Here's how the part is built. I have some questions about the finished solid (model axes, mm). Face numbers are marked on the shaded views. A direction names the side the tool comes from. Give positions to 0.01 mm unless a question says otherwise; leave off trailing zeros. Loops run counter-clockwise (first coordinate to the right, second up) from the corner with the lowest first, then second, coordinate; pieces in that order, holes last. Notation, with made-up numbers: M -31.5,-37 L 22.5,-37 A25 cw 22.5,-7 Z; hole C 13.5,44 d3. An arc over 180 degrees is marked long. Answer as CSV lines item,"result". Start each with the question number.
Item 1: If I drill on line 1 along X through (y, z) = (0, -20.5); line 2 along Z through (x, y) = (10.5, -3.5); line 3 along Z through (x, y) = (4, 6.5), over which ranges is the centre line in solid material (lowest first)? Write a range as from..to.
Item 2: I want a section at B-B on z = -4. List the corners of the cut face in (x, y) for me, plus the area to 3 significant figures.
Item 3: I want a section at C-C on x = 13. List the corners of the cut face in (y, z) for me.
Item 4: I want a section at A-A on y = 0. List the corners of the cut face in (x, z) for me.
Item 5: If we mould it in two halves opening along Y, with no side actions, what happens to the marked faces 1, 2, 3 and 4? For each: released by +Y, released by -Y, zero draft, split by the parting line, or undercut.
Item 6: For the marked faces 5, 6 and 7, which set-ups out of +Z, -Z, +X, -X, +Y, -Y let a thin tool reach every point of the face, with its end or its side?
Item 7: I want a section at D-D on z = 12.5. List the corners of the cut face in (x, y) for me, plus the area to 3 significant figures.
Item 8: Will these pins go through, and if not, where does the flat tip stop? P1, Ø4, axis at y = 19.05, z = 0, coming from the +X side; P2, Ø2, axis at x = 16, y = 0, coming from the +Z side; P3, Ø6, axis at x = 14, y = -6, coming from the +Z side; P4, Ø4, axis at y = 9, z = 7, coming from the -X side.
Autodesk Inventor part; units mm, degrees
ref_plane "YZ Plane" through (0, 0, 0) normal (1, 0, 0) x (0, 1, 0)
ref_plane "XZ Plane" through (0, 0, 0) normal (0, 1, 0) x (-1, 0, 0)
ref_plane "XY Plane" through (0, 0, 0) normal (0, 0, 1) x (1, 0, 0)
sketch "Sketch1" plane through (0, 0, 0) normal (1, 0, 0) x (0, 1, 0)
  circle A0 centre (0, 0) radius 15
  line L0 (0, 0) -> (7.5, 0)
  line L1 (7.5, 0) -> (3.75, -6.4952)
  line L2 (3.75, -6.4952) -> (-3.75, -6.4952)
  line L3 (-3.75, -6.4952) -> (-7.5, 0)
  line L4 (-7.5, 0) -> (-3.75, 6.4952)
  line L5 (-3.75, 6.4952) -> (3.75, 6.4952)
  line L6 (3.75, 6.4952) -> (7.5, 0)
  dimension "d0" = 30
  dimension "d1" = 7.5
extrude "Extrusion1" add sketch "Sketch1" along normal blind 32.75
sketch "Sketch2" plane through (0, 0, 0) normal (-1, 0, 0) x (0, 0, 1)
  circle A0 centre (0, 0) radius 22.5
  line L0 (0, 7.5) -> (-6.4952, 3.75)
  line L1 (-6.4952, 3.75) -> (-6.4952, -3.75)
  line L2 (-6.4952, -3.75) -> (0, -7.5)
  line L3 (0, -7.5) -> (6.4952, -3.75)
  line L4 (6.4952, -3.75) -> (6.4952, 3.75)
  line L5 (6.4952, 3.75) -> (0, 7.5)
  dimension "d4" = 45
extrude "Extrusion2" add sketch "Sketch2" against normal blind 5
sketch "Sketch3" plane through (0, 0, 0) normal (-1, 0, 0) x (0, 0, 1)
  circle A0 centre (0, 19.05) radius 1.45
  circle A1 centre (-16.4978, -9.525) radius 1.45
  circle A2 centre (16.4978, -9.525) radius 1.45
  point P0 (0, 0)
  dimension "d11" = 360
extrude "Extrusion3" cut sketch "Sketch3" against normal up to surface (5 mm away)
sketch "Sketch4" plane through (0, 0, 0) normal (-1, 0, 0) x (0, 0, 1)
  line L0 (6.4952, 3.75) -> (0, 7.5)
  circle A0 centre (0, 0) radius 7.5
properties part number "wheel_gearing_mount_long"
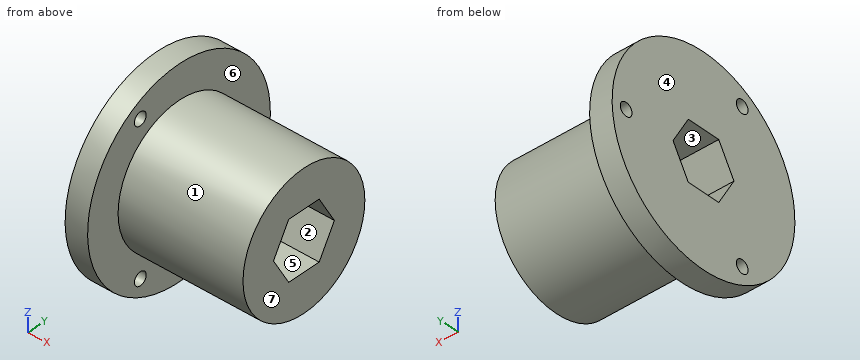
Result:
1,line 1,"0..5"
1,line 2,"-14.59..-6.5, 6.5..14.59"
1,line 3,"-21.54..-1.73, 1.73..21.54"
2,outline,"M 0,-22.14 L 5,-22.14 L 5,-14.46 L 32.75,-14.46 L 32.75,-5.19 L 0,-5.19 Z; M 0,5.19 L 32.75,5.19 L 32.75,14.46 L 5,14.46 L 5,22.14 L 0,22.14 Z"
2,area,"684 mm^2"
3,outline,"C 0,0 d30; hole M -7.5,0 L -3.75,-6.5 L 3.75,-6.5 L 7.5,0 L 3.75,6.5 L -3.75,6.5 Z"
4,outline,"M 0,-22.5 L 5,-22.5 L 5,-15 L 32.75,-15 L 32.75,-6.5 L 0,-6.5 Z; M 0,6.5 L 32.75,6.5 L 32.75,15 L 5,15 L 5,22.5 L 0,22.5 Z"
5,face 1,"split by the parting line"
5,face 2,"undercut"
5,face 3,"undercut"
5,face 4,"zero draft"
6,face 5,"+X, -X"
6,face 6,"+X"
6,face 7,"+Z, -Z, +X, +Y, -Y"
7,outline,"M 0,-18.71 L 5,-18.71 L 5,-8.29 L 32.75,-8.29 L 32.75,8.29 L 5,8.29 L 5,18.71 L 0,18.71 Z"
7,area,"647 mm^2"
8,P1,"x = 5"
8,P2,"z = 15"
8,P3,"z = 14.7"
8,P4,"x = 0"
